from build123d import *

# Parameters (mm, degrees)
SKETCH1_R            = 15
BOSS_EXTRUDE2_DEPTH  = 5
SKETCH10_R           = 0.026716532
BOSS_EXTRUDE10_DEPTH = 10
BOSS_EXTRUDE13_START = 1
SKETCH12_R           = 15
BOSS_EXTRUDE13_DEPTH = 1
BOSS_EXTRUDE14_START = 20
BOSS_EXTRUDE14_DEPTH = 20


with BuildPart() as part:
    # Sketch1 → Boss-Extrude2 (new body)
    with BuildSketch(Plane.XY):
        with Locations((0.153154005, 2.896729922)):
            Circle(SKETCH1_R)
        with BuildLine():
            Line((-3.858366409, 8.353410796), (-3.858366409, 15.623324251))
            ThreePointArc((-3.858366409, 15.623324251), (0.153154005, 16.236968805), (4.164674419, 15.623324251))
            Line((4.164674419, 15.623324251), (4.164674419, 8.353410796))
            ThreePointArc((4.164674419, 8.353410796), (0.153154005, 9.669296806), (-3.858366409, 8.353410796))
        make_face(mode=Mode.SUBTRACT)
        with BuildLine():
            Line((-3.858366409, -2.559950952), (-3.858366409, -9.987163584))
            ThreePointArc((-3.858366409, -9.987163584), (0.153154005, -10.600808139), (4.164674419, -9.987163584))
            Line((4.164674419, -9.987163584), (4.164674419, -2.559950952))
            ThreePointArc((4.164674419, -2.559950952), (0.153154005, -3.875836962), (-3.858366409, -2.559950952))
        make_face(mode=Mode.SUBTRACT)
    extrude(amount=BOSS_EXTRUDE2_DEPTH)

    # Sketch10 → Boss-Extrude10 (add)
    with BuildSketch(Plane.XY.offset(5)):
        with BuildLine():
            Line((-2.094128576, 16.047452534), (-2.094128576, 17.727431895))
            ThreePointArc((-2.094128576, 17.727431895), (-9.62669163, -8.476687302), (15.153154005, 2.896729922))
            ThreePointArc((15.153154005, 2.896729922), (11.304753393, 12.928770148), (1.734243192, 17.813169074))
            Line((1.734243192, 17.813169074), (1.734243192, 16.14349683))
            ThreePointArc((1.734243192, 16.14349683), (2.961528164, 15.939802873), (4.164674419, 15.623324251))
            ThreePointArc((4.164674419, 15.623324251), (13.572042477, 2.818080333), (4.164674419, -9.987163584))
            ThreePointArc((4.164674419, -9.987163584), (0.153154005, -10.600808139), (-3.858366409, -9.987163584))
            ThreePointArc((-3.858366409, -9.987163584), (-13.265734467, 2.818080333), (-3.858366409, 15.623324251))
            ThreePointArc((-3.858366409, 15.623324251), (-2.983424534, 15.865242588), (-2.094128576, 16.047452534))
        make_face()
        with Locations((10.491847297, -7.276178058)):
            Circle(SKETCH10_R, mode=Mode.SUBTRACT)
    extrude(amount=BOSS_EXTRUDE10_DEPTH)

    # Sketch12 → Boss-Extrude13 (add)
    with BuildSketch(Plane(origin=(0, 0, 0), x_dir=(-1, 0, 0), z_dir=(0, 0, -1)).offset(BOSS_EXTRUDE13_START)):
        with Locations((-0.153154005, 2.896729922)):
            Circle(SKETCH12_R)
    extrude(amount=-BOSS_EXTRUDE13_DEPTH)

    # Sketch13 → Boss-Extrude14 (add)
    with BuildSketch(Plane(origin=(0, 0, -1), x_dir=(-1, 0, 0), z_dir=(0, 0, -1)).offset(BOSS_EXTRUDE14_START)):
        with BuildLine():
            ThreePointArc((9.596845995, 2.896729922), (-5.50307382, -5.254396256), (-4.032047949, 11.841934323))
            Line((-4.032047949, 11.841934323), (-4.032047949, 17.386525703))
            ThreePointArc((-4.032047949, 17.386525703), (-9.285968216, -9.002501338), (14.846845995, 2.896729922))
            ThreePointArc((14.846845995, 2.896729922), (11.746077255, 12.029544133), (3.725739939, 17.386525703))
            Line((3.725739939, 17.386525703), (3.725739939, 11.841934323))
            ThreePointArc((3.725739939, 11.841934323), (7.997972173, 8.246649737), (9.596845995, 2.896729922))
        make_face()
    extrude(amount=-BOSS_EXTRUDE14_DEPTH)


solid = part.part
Source: CAD feature listing. Evaluate the final solid. Frame: model axes, mm. A direction names the side the tool comes from. Round coordinates to 2 decimals unless told otherwise and drop trailing zeros. Loops run counter-clockwise (first coordinate to the right, second up) from the corner with the lowest first, then second, coordinate; pieces in that order, holes last. Notation, with made-up numbers: (5.25, -9) -> (10.25, -9) arc R5 cw to (10.25, -1) -> close; hole circle Ø3 at (86.25, -16.75). An arc over 180 degrees is marked (long way). Answer as a JSON object with one key per item and string values. Group by question number.
Q1. Section query B-B (y = -1.75). Output: boundary loops of the cut face in (x, z).
Q2. Contact query for flat-ended pins moving along their axis: P1, Ø1.5, axis at y = -7.5, z = -17, coming from the -X side; P2, Ø7.5, axis at x = 6, y = 0.5, coming from the +Z side; P3, Ø1, axis at x = 3, z = -1, coming from the -Y side. Output: stop coordinate, or through.
Q3. Access query for faces 1 (the flat face through (-9, 13, 15)), 2 (the flat face through (-2.094, 17, 10)), 3 (the flat face through (4.032, 15, -11)), 4 (the flat face through (4.165, 12, 2)). Directions: +Z, -Z, +X, -X, +Y, -Y. A direction counts if a zero-diameter tool reaches every point of the face in a straight line with its end or side. Return the directions, or none.
Q4. Section query C-C (x = -4.5). Output: boundary loops of the cut face in (y, z).
Q5. Section query A-A (z = 2). Output: boundary loops of the cut face in (x, y), plus the area to 3 significant figures.
Q6. Mould query, pull axis Y, two halves, no side actions, for faces 5 (the flat face through (0, 3, -1)), 6 (the flat face through (-3, -7, -21)). Classes: pulls with the +Y half, pulls with the -Y half, needs draft (parallel to the pull), parting line crosses it, or undercut.
Q7. Section query D-D (z = 12.5). Output: boundary loops of the cut face in (x, y), plus the area to 3 significant figures.
Q8. Ray query, line 1 (Y direction, x = 2, z = 4); line 2 (Y direction, x = 2.5, z = 1); line 3 (X direction, y = 14, z = -19). Return the intervals inside material, ascending. Write a range as from..to.
Completed:
{
 "1": {"outline": "(-14.11, -21) -> (-8.42, -21) -> (-8.42, -1) -> (8.72, -1) -> (8.72, -21) -> (14.42, -21) -> (14.42, 15) -> (12.77, 15) -> (12.77, 5) -> (-12.46, 5) -> (-12.46, 15) -> (-14.11, 15) -> close"},
 "2": {"P1": "x = -11.33", "P2": "z = 5", "P3": "y = -11.92"},
 "3": {"face 1": "+Z, +X, -X, +Y, -Y", "face 2": "+Z, +Y", "face 3": "-Z, +Y", "face 4": "+Z"},
 "4": {"outline": "(-11.36, -21) -> (-5.67, -21) -> (-5.67, -1) -> (11.46, -1) -> (11.46, -21) -> (17.16, -21) -> (17.16, 15) -> (15.4, 15) -> (15.4, 5) -> (-9.77, 5) -> (-9.77, 15) -> (-11.36, 15) -> close"},
 "5": {"outline": "circle Ø30 at (0.15, 2.9); hole (-3.86, -9.99) arc R13.42 ccw to (4.16, -9.99) -> (4.16, -2.56) arc R6.77 cw to (-3.86, -2.56) -> close; hole (-3.86, 8.35) arc R6.77 cw to (4.16, 8.35) -> (4.16, 15.62) arc R13.42 ccw to (-3.86, 15.62) -> close", "area": "597 mm²"},
 "6": {"face 5": "undercut", "face 6": "needs draft"},
 "7": {"outline": "(-2.09, 16.05) -> (-2.09, 17.73) arc R15 ccw (long way) to (1.73, 17.81) -> (1.73, 16.14) arc R13.42 cw (long way) to start; hole circle Ø0.05 at (10.49, -7.28)", "area": "135 mm²"},
 "8": {"line 1": "-11.99..-10.47, -3.62..9.41, 16.11..17.78", "line 2": "-11.92..-10.39, -3.46..9.25, 16.03..17.71", "line 3": "-9.93..-3.73, 4.03..10.24"}
}
